Geometry: see drawing. Coordinates: mm, zero at the bounding-box minimum. A direction names the side the tool comes from. Coordinates: 2 decimals unless noted, no trailing zeros. Loops run counter-clockwise (first coordinate to the right, second up) from the corner with the lowest first, then second, coordinate; pieces in that order, holes last. Notation, with made-up numbers: (51.25, 61) - (82.25, 61) arc R25 ccw to (82.25, 100) - close; hole circle Ø6 at (64.5, 57.5). An arc over 180 degrees is marked (long way). Use one line per item in the form item = value.
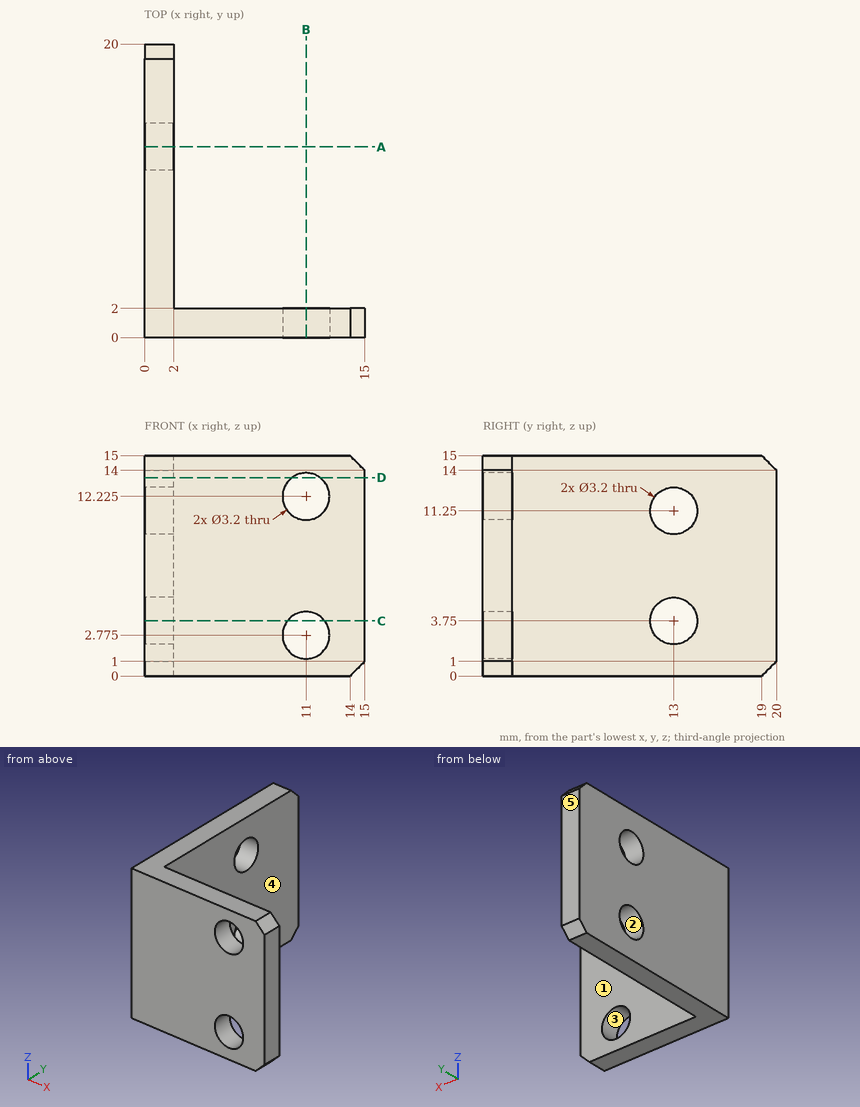
Q1. Cut plane C-C, the plane z = 3.75. Return loops of the section in (x, y).
Check values:
outline = (0, 0) - (9.73, 0) - (9.73, 2) - (2, 2) - (2, 11.4) - (0, 11.4) - close; (0, 14.6) - (2, 14.6) - (2, 20) - (0, 20) - close; (12.27, 0) - (15, 0) - (15, 2) - (12.27, 2) - close
Q2. Set-up query: the marked faces 1 and 2. Return all of +Z, -Z, +X, -X, +Y, -Y with unobstructed straight access to the full face (end or side cutting, diameter ignored); none if empty.
Check values:
face_1 = +Z, -Z, +X, +Y
face_2 = +X, -X
Q3. Cut plane B-B, the plane x = 11. Return loops of the section in (y, z) (3 decimals), then the cut area to 3 significant figures.
Check values:
outline = (0, 0) - (2, 0) - (2, 1.175) - (0, 1.175) - close; (0, 4.375) - (2, 4.375) - (2, 10.625) - (0, 10.625) - close; (0, 13.825) - (2, 13.825) - (2, 15) - (0, 15) - close
area = 17.2 mm²
Q4. Pull-direction query (X, two-part tool) for the marked faces 3, 4 and 5; classes: pulls with the +X half, pulls with the -X half, needs draft (parallel to the pull), parting line crosses it, or undercut.
Check values:
face_3 = undercut
face_4 = pulls with the +X half
face_5 = needs draft
Q5. Cut plane D-D, the plane z = 13.5. Return loops of the section in (x, y).
Check values:
outline = (0, 0) - (10.03, 0) - (10.03, 2) - (2, 2) - (2, 20) - (0, 20) - close; (11.97, 0) - (15, 0) - (15, 2) - (11.97, 2) - close
Q6. Ray query, line 1 along Z through (x, y) = (11, 1.35) (3 decimals); line 2 along Y through (x, z) = (1.25, 3.75); line 3 along X through (y, z) = (16, 10.75). Return the intervals inside material, ascending. Write a range as [from, to].
Check values:
line_1 = [0, 1.175], [4.375, 10.625], [13.825, 15]
line_2 = [0, 11.4], [14.6, 20]
line_3 = [0, 2]
Q7. Cut plane A-A, the plane y = 13. Return loops of the section in (x, z).
Check values:
outline = (0, 0) - (2, 0) - (2, 2.15) - (0, 2.15) - close; (0, 5.35) - (2, 5.35) - (2, 9.65) - (0, 9.65) - close; (0, 12.85) - (2, 12.85) - (2, 15) - (0, 15) - close
Q8. First-contact query: P1, Ø4, axis at y = 11, z = 8, coming from the -X side; P2, Ø8, axis at x = 8, z = 3, coming from the +Y side; P3, Ø4, axis at y = 13, z = 11.25, coming from the +X side. Flat tips, straight axial feed; report the tip coordinate or a pass-through.
Check values:
P1 = 0
P2 = 2
P3 = 2
